Input: part model. Units: mm. Frame: model coordinates. Face numbers are marked on the shaded views. A direction names the side the tool comes from. Give positions to 0.01 mm unless a question says otherwise; leave off trailing zeros. Order: outer loops, then holes, each group sorted by start corner. A loop starts at its lowest first (then second) coordinate and runs counter-clockwise, first axis right, second up. Notation, with made-up numbers: (50.25, 27.5) - (57.25, 27.5) arc R30 ccw to (57.25, 53.5) - close; hole circle Ø10 at (30, -14.5). An arc over 180 degrees is marked (long way). Answer in a Markdown table with one row per item. Add a question column.
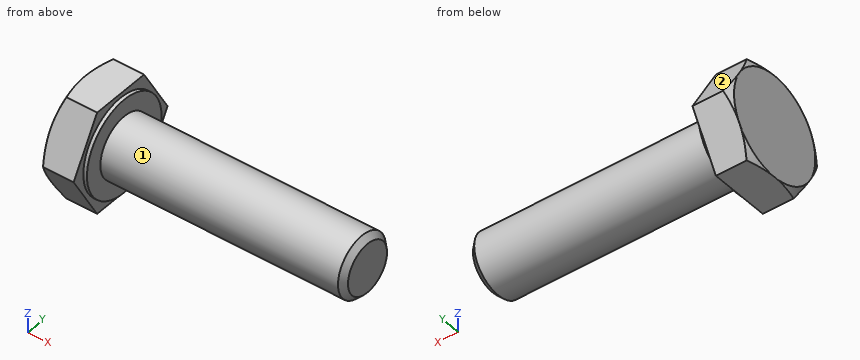
Autodesk Inventor part; units mm, degrees
ref_plane "Work Plane1" through (1.525, 0, 0) normal (0, 0, 1) x (1, 0, 0)
ref_plane "YZ Plane" through (0, 0, 0) normal (1, 0, 0) x (0, 1, 0)
ref_plane "XZ Plane" through (0, 0, 0) normal (0, 1, 0) x (-1, 0, 0)
sketch "Sketch1" plane through (0, 0, 0) normal (0, 0, 1) x (1, 0, 0)
  line L0 (0, 7.8) -> (0, 5)
  line L1 (14, 5) -> (40, 5)
  line L2 (40, 5) -> (40, 0)
  line L3 (40, 0) -> (-0.6001, 0)
  line L4 (-8.7201, 0) -> (48.12, 0)
  line L5 (-0.6001, 0) -> (-0.6001, 7.8)
  line L6 (-0.6001, 7.8) -> (0, 7.8)
  line L7 (14, 5) -> (13.0797, 5)
  line L8 (13.0797, 5) -> (0, 5)
  line L9 (0, -1.56) -> (0, 9.36)
  dimension "d0" = 40
  dimension "d1" = 26
  dimension "d2" = 10
  dimension "d9" = 0.6001
  dimension "d10" = 15.6
  dimension "d13" = 0.9203
  dimension "d14" = 10
revolve "Body" add sketch "Sketch1" angle 360 about axis through (40, 0, 0) along (-1, 0, 0)
sketch "Sketch2" plane through (-0.6001, 0, 0) normal (-1, 0, 0) x (0, 0, 1)
  line L0 (0, 9.815) -> (8.5, 4.9075)
  line L1 (8.5, 4.9075) -> (8.5, -4.9075)
  line L2 (8.5, -4.9075) -> (0, -9.815)
  line L3 (0, -9.815) -> (-8.5, -4.9075)
  line L4 (-8.5, -4.9075) -> (-8.5, 4.9075)
  line L5 (-8.5, 4.9075) -> (0, 9.815)
  point P0 (0, 0)
  point P1 (0, 0)
  dimension "d11" = 17
extrude "Head" add sketch "Sketch2" along normal blind 5.8
sketch "Sketch4" plane through (0, 0, 0) normal (0, 0, 1) x (1, 0, 0)
  line L0 (-6.4001, 8.5) -> (-6.4001, 9.815)
  line L1 (-6.4001, 9.815) -> (-5.6409, 9.815)
  line L2 (-5.6409, 9.815) -> (-6.4001, 8.5)
  line L3 (-7.5601, 0) -> (0.5599, 0)
  line L4 (-0.6001, 9.815) -> (-6.4001, 9.815)
  line L5 (-6.4001, 4.9075) -> (-6.4001, 9.815)
  dimension "d5" = 30
  dimension "d19" = 17
revolve "Chamfer1" cut sketch "Sketch4" angle 360 about axis through (-10, 0, 0) along (1, 0, 0)
thread "Thread"
chamfer "Chamfer2" distance 0.9202 distance2 0.9203 1 edges at (40, -5, 0) measured on face at (40, 1.2281, 0.495)
ref_plane "Work Plane1" through (1.525, 0, 0) normal (0, 0, 1) x (1, 0, 0)
equation "\"d0\" = NLG"
equation "\"d1\" = GEL"
equation "\"d2\" = GD"
equation "\"d10\" = SD2"
equation "\"d14\" = BDM"
equation "\"d11\" = SW"
equation "\"d3\" = KOH - SD"
equation "\"d5\" = ANG1"
equation "\"d19\" = SW0"
equation "\"d15\" = GEL"
equation "\"d6\" = -0.5 * SPD + 0.5 * GD"
equation "\"NLG\" = 40"
equation "\"GD\" = NND"
equation "\"BDM\" = NND"
equation "\"KOH\" = 6.4"
equation "\"GEL\" = 26"
equation "\"SW\" = 17"
equation "\"SW0\" = SW"
equation "\"SPD\" = NND - 1.2269 * PTC"
equation "\"SD2\" = 15.6"
equation "\"SD\" = 0.6"
equation "\"ANG1\" = 30deg"
equation "\"GAL\" = 0.61345 * PTC"
equation "\"GUL\" = 0.61345 * PTC"
equation "\"RR\" = 0.4"
equation "\"GD1\" = THREADDIA - 1.2269 * PTC"
equation "\"TOA\" = 30deg"
equation "\"PTC\" = 1.5"
equation "\"E0\" = 1.155 * SW"
properties part number "DIN 931-1 - M10 x 40" material "Steel, Mild"
Q1. Access query for the marked faces 1 and 2. Directions: +Z, -Z, +X, -X, +Y, -Y. A direction counts if a zero-diameter tool reaches every point of the face in a straight line with its end or side. Return the directions, or none.
Q2. Section A-A, the plane x = 13.5. Return loops of the section in (y, z).
Q3. Line query: probe 1 along X at (y, z) = (-4, 7.5); probe 2 along X at (y, z) = (-6.75, 3.5); probe 3 along Z at (x, y) = (12, -1). Output: solid intervals per line, ascending.
Q4. Contact query for flat-ended pins moving along their axis: P1, Ø6, axis at x = 7.5, y = 7.5, coming from the +Z side; P2, Ø1.5, axis at x = 32.5, y = 3.5, coming from the +Z side; P3, Ø4, axis at x = 12.5, z = -1, coming from the -Y side; P4, Ø1.5, axis at x = 12, y = 6, coming from the +Z side. Output: stop coordinate, or through.
Computed:
| question | item | result |
|---|---|---|
| 1 | face 1 | +X |
| 1 | face 2 | +Z, +X, -X, +Y |
| 2 | outline | circle Ø10 at (0, 0) |
| 3 | probe 1 | x = -6.4 to -0.6 |
| 3 | probe 2 | x = -6.4 to 0 |
| 3 | probe 3 | z = -4.9 to 4.9 |
| 4 | P1 | stops at z = 2.18 |
| 4 | P2 | stops at z = 4.18 |
| 4 | P3 | stops at y = -5 |
| 4 | P4 | passes through |
